from build123d import *

# Parameters (mm, degrees)
F0_R     = 70.754206
F0_R_2   = 30.61563
F1_DEPTH = 62.94323
F2_SIZE  = 5.08
F3_R     = 49.110823
F4_DEPTH = 31.93714
F5_R     = 30.807574
F6_DEPTH = 25.4


with BuildPart() as f1:
    # F0 (on Front) → F1 (new body)
    with BuildSketch(Plane.XZ):
        Circle(F0_R)
        Circle(F0_R_2, mode=Mode.SUBTRACT)
    extrude(amount=F1_DEPTH)

    # F2
    f2_edges = [f1.edges().sort_by_distance(p)[0] for p in [
        (-70.754206, -62.94323, 0),
        (-30.61563, -62.94323, 0),
        (-70.754206, 0, 0),
        (-30.61563, 0, 0),
    ]]
    chamfer(f2_edges, length=F2_SIZE)

    # F3 (on face) → F4 (join)
    with BuildSketch(Plane(origin=(0, 0, 0), x_dir=(-1, 0, 0), z_dir=(0, 1, 0))):
        Circle(F3_R)
    extrude(amount=F4_DEPTH)

    # F5 (on Front) → F6 (join)
    with BuildSketch(Plane.XZ):
        Circle(F5_R)
    extrude(amount=F6_DEPTH)


solid = f1.part
For this review, take the finished solid that the model builds, in its own axes (mm). A direction names the side the tool comes from. Coordinates: 2 decimals unless noted, no trailing zeros. Loops run counter-clockwise (first coordinate to the right, second up) from the corner with the lowest first, then second, coordinate; pieces in that order, holes last. Notation, with made-up numbers: (88.5, -22.5) - (96.5, -22.5) arc R20 ccw to (96.5, -8.5) - close; hole circle Ø11 at (35.25, 52.5). An arc over 180 degrees is marked (long way). Use a Markdown table: item, result. Add a question column.
Item 1: We need section D-D (y = -12). Give the boundary of the cut face in (x, z).
Item 2: We need section B-B (x = 0). Give the boundary of the cut face in (y, z).
Item 3: We need section C-C (y = -49.5). Give the boundary of the cut face in (x, z).
Item 4: Tool access review of faces 1 (the face through (0, -25.4, 0)), 2 (the face through (-46.843, 15.745, 14.752)), 3 (the face through (27, 0, -16)): name each direction out of +Z, -Z, +X, -X, +Y, -Y from which nothing blocks a thin tool from reaching the whole face with its end or side.
Item 5: Insertion check: pin 1 Ø1.5 at (y, z) = (-51.5, 18.5) entering from +X; pin 2 Ø3 at (y, z) = (-35.5, 33.5) entering from -X; pin 3 Ø18.5 at (x, z) = (4.5, 5) entering from -Y. Each pin has a flat end and moves straight along its axis. Give the tip position at first contact, or say it passes through.
Item 6: Mouldability with a two-part tool opening along X and no side actions: class faces 4 (the face through (29.385, -2.41, 9.254)), 5 (the face through (62.88, -0.25, 19.8)), 6 (the face through (28, -62.943, -28)) as pulls with the +X half, pulls with the -X half, needs draft (parallel to the pull), parting line crosses it, or undercut.
Item 7: We need section A-A (z = 0). Give the boundary of the cut face in (x, y), and give its area (3 significant figures).
Item 8: For line 1 (Z direction, x = 0, y = -40); line 2 (Y direction, x = -61.5, z = -18); line 3 (X direction, y = -34, z = 61.5), list the stretches that pass through material, from the lowest coordinate up.
Results list:
| question | item | result |
|---|---|---|
| 1 | outline | circle Ø141.51 at (0, 0) |
| 2 | outline | (-62.94, -65.67) - (-57.86, -70.75) - (-5.08, -70.75) - (0, -65.67) - (0, -49.11) - (31.94, -49.11) - (31.94, 49.11) - (0, 49.11) - (0, 65.67) - (-5.08, 70.75) - (-57.86, 70.75) - (-62.94, 65.67) - (-62.94, 35.7) - (-57.86, 30.62) - (-25.4, 30.62) - (-25.4, -30.62) - (-57.86, -30.62) - (-62.94, -35.7) - close; hole (-4.89, -30.81) - (0, -35.7) - (0, -30.81) - close; hole (-4.89, 30.81) - (0, 30.81) - (0, 35.7) - close |
| 3 | outline | circle Ø141.51 at (0, 0); hole circle Ø61.23 at (0, 0) |
| 4 | face 1 | -Y |
| 4 | face 2 | +Y |
| 4 | face 3 | none |
| 5 | pin 1 | stops at x = 68.49 |
| 5 | pin 2 | stops at x = -63.1 |
| 5 | pin 3 | stops at y = -25.4 |
| 6 | face 4 | undercut |
| 6 | face 5 | parting line crosses it |
| 6 | face 6 | needs draft |
| 7 | outline | (-70.75, -57.86) - (-65.67, -62.94) - (-35.7, -62.94) - (-30.62, -57.86) - (-30.62, -25.4) - (30.62, -25.4) - (30.62, -57.86) - (35.7, -62.94) - (65.67, -62.94) - (70.75, -57.86) - (70.75, -5.08) - (65.67, 0) - (49.11, 0) - (49.11, 31.94) - (-49.11, 31.94) - (-49.11, 0) - (-65.67, 0) - (-70.75, -5.08) - close; hole (-35.7, 0) - (-30.81, -4.89) - (-30.81, 0) - close; hole (30.81, -4.89) - (35.7, 0) - (30.81, 0) - close |
| 7 | area | 9,640 mm^2 |
| 8 | line 1 | z = -70.75 to -30.62, 30.62 to 70.75 |
| 8 | line 2 | y = -62.94 to 0 |
| 8 | line 3 | x = -34.98 to 34.98 |
